Autodesk Inventor part; units mm, degrees
ref_plane "Arbeitsebene3" through (7, 0, 0) normal (1, 0, 0) x (0, 1, 0)
ref_plane "Arbeitsebene4" through (0, 7, 0) normal (0, 1, 0) x (-1, 0, 0)
ref_plane "XY Plane" through (0, 0, 0) normal (0, 0, 1) x (1, 0, 0)
sketch "Skizze1" plane through (0, 0, 0) normal (0, 0, 1) x (1, 0, 0)
  circle A0 centre (0, 0) radius 7
  dimension "d0" = 14
extrude "Extrusion1" add sketch "Skizze1" along normal blind 25
sketch "Skizze2" plane through (0, 0, 25) normal (0, 0, 1) x (1, 0, 0)
  circle A0 centre (0, 0) radius 7
hole "Bohrung1" at (0, 0, 25) direction (0, 0, -1) diameter 4.134 depth 11.5 tip angle 118
chamfer "Fasen1" distance 1 angle 45 1 edges at (0, 2.067, 25)
ref_plane "Arbeitsebene1" through (-7, 0, 0) normal (1, 0, 0) x (0, 1, 0)
ref_plane "Arbeitsebene2" through (0, -7, 0) normal (0, 1, 0) x (-1, 0, 0)
ref_plane "Arbeitsebene3" through (7, 0, 0) normal (1, 0, 0) x (0, 1, 0)
sketch "Skizze6" plane through (7, 0, 0) normal (1, 0, 0) x (0, 1, 0)
  line L0 (-7, 0) -> (-7, 25)
  line L1 (7, 0) -> (7, 25)
  line L2 (-7, 5) -> (7, 5)
  line L3 (7, 5) -> (7, 15)
  line L4 (7, 15) -> (-7, 15)
  line L5 (-7, 15) -> (-7, 5)
  line L6 (7, 25) -> (-7, 25)
  point P0 (0, 0)
  point P1 (-7, 15)
  point P2 (7, 5)
  dimension "d29" = 10
  dimension "d30" = 10
extrude "Extrusion4" cut sketch "Skizze6" against normal blind 2 contours L0 L4 L1 L2
sketch "Skizze7" plane through (5, 0, 0) normal (1, 0, 0) x (0, 0, -1)
  line L0 (-5, -4.899) -> (-5, 4.899)
  line L1 (0, 7) -> (0, -7)
  point P0 (0, 0)
  point P1 (-10, 0)
  point P2 (0, 0)
  point P3 (0, 0)
  point P4 (0, 0)
  dimension "d33" = 5
hole "Bohrung3" at (5, 0, 10) direction (-1, 0, 0) diameter 4.134 end through all
ref_plane "Arbeitsebene4" through (0, 7, 0) normal (0, 1, 0) x (-1, 0, 0)
sketch "Skizze8" plane through (0, 7, 0) normal (0, 1, 0) x (-1, 0, 0)
  line L0 (-5, 5) -> (-5, 5)
  line L1 (-5, 7.933) -> (-5, 12.067)
  line L2 (-5, 5) -> (-5, 15)
  line L3 (-5, 15) -> (-5, 5)
  line L4 (-5, 15) -> (-7, 15)
  line L5 (-5, 15) -> (-5, 5)
  line L6 (-5, 5) -> (-5, 15)
  line L7 (-5, 15) -> (-5, 15)
  line L8 (-7, 5) -> (-5, 5)
  line L9 (-5, 5) -> (-7, 3)
  line L10 (-7, 0) -> (-7, 25)
  line L11 (-5, 5) -> (-2.1716, 5) construction
  line L12 (-7, 3) -> (-7, 5)
  line L13 (-5, 15) -> (-7, 17)
  line L14 (-5, 15) -> (-2.1716, 15) construction
  line L15 (-7, 17) -> (-7, 15)
  point P0 (0, 0)
  point P1 (-5, 24.433)
  point P2 (-5, 28.567)
  dimension "d42" = 135
  dimension "d43" = 135
extrude "Extrusion5" cut sketch "Skizze8" against normal through all contours L9 L10 L8 | L4 L10 L13
properties part number "TS_V1_Fallmagazin_Schieberanbindung_int"
The listing builds one solid part. Answer for the finished solid, in the listing's coordinates (mm). A direction names the side the tool comes from. Coordinates: 2 decimals unless noted, no trailing zeros. Write each loop counter-clockwise with the first axis right and the second up, starting at its lowest first coordinate (ties: lowest second). Pieces come first, ordered by that corner, then holes. Notation, with made-up numbers: (-16, 83) - (21, 83) arc R33 ccw to (21, 119) - close; hole circle Ø8 at (78, 51.25). An arc over 180 degrees is marked (long way). Put each result on its own line as item: value.
1. The part is cut by section B-B on z = 2.25. Give the vertices of the cut face in (x, y).
Answer sheet:
outline: circle Ø14 at (0, 0)
2. A tool of negligible diameter and unlimited length cuts with its end or side. For faces 1 (the face through (-1.085, -0.091, 12.065)), 2 (the face through (1.26, 1.64, 18.68)), 3 (the face through (6, 0, 16)), from which of +Z, -Z, +X, -X, +Y, -Y can it reach the whole face along a straight path? Write none if from no direction.
Answer sheet:
face 1: +X, -X
face 2: +Z
face 3: +X, +Y, -Y
3. Determine the mould class of faces 4 (the face through (-0.137, -0.332, 12.474)), 5 (the face through (-6.993, -0.308, 12.325)), 6 (the face through (1.5, -3, 25)) for opening direction X: pulls with the +X half, pulls with the -X half, needs draft (parallel to the pull), parting line crosses it, or undercut.
Answer sheet:
face 4: undercut
face 5: parting line crosses it
face 6: needs draft
4. The part is cut by section A-A on z = 10. Give the vertices of the cut face in (x, y).
Answer sheet:
outline: (-6.69, -2.07) arc R7 ccw to (5, -4.9) - (5, -2.07) - close; (-6.69, 2.07) - (5, 2.07) - (5, 4.9) arc R7 ccw to start
5. The part is cut by section D-D on y = -5.25. Give the vertices of the cut face in (x, z).
Answer sheet:
outline: (-4.63, 0) - (4.63, 0) - (4.63, 25) - (-4.63, 25) - close
6. Flat-ended cylindrical pins translate along their axes: pin 1 Ø5 at (y, z) = (0, 11) entering from +X; pin 2 Ø1.5 at (x, z) = (4, 11.5) entering from +Y; pin 3 Ø1 at (y, z) = (5, 11.5) entering from -X; pin 4 Ø8 at (x, z) = (-3, 18.5) entering from +Y. Find the tip coordinate at first contact, or state that the pin passes through.
Answer sheet:
pin 1: stops at x = 5
pin 2: stops at y = 6.2
pin 3: stops at x = -5.36
pin 4: stops at y = 7
7. Find the intervals of material crossed by line 1 along Y through (x, z) = (0, 18.75); line 2 along Y through (x, z) = (1, 10), in increasing order. Write a range as from..to.
Answer sheet:
line 1: y = -7..-2.07, 2.07..7
line 2: y = -6.93..-2.07, 2.07..6.93
8. The part is cut by section C-C on z = 20.5. Give the vertices of the cut face in (x, y).
Answer sheet:
outline: circle Ø14 at (0, 0); hole circle Ø4.13 at (0, 0)
